Print and shaded views of the part. All mm, measured from the part's lowest x, y and z. A direction names the side the tool comes from. Round coordinates to 2 decimals unless told otherwise and drop trailing zeros. Loops run counter-clockwise (first coordinate to the right, second up) from the corner with the lowest first, then second, coordinate; pieces in that order, holes last. Notation, with made-up numbers: (72, 32) - (126, 32) arc R33 cw to (126, 66) - close; hole circle Ø9 at (16.25, -39). An arc over 180 degrees is marked (long way). Answer as a JSON object with one key per item and string values.
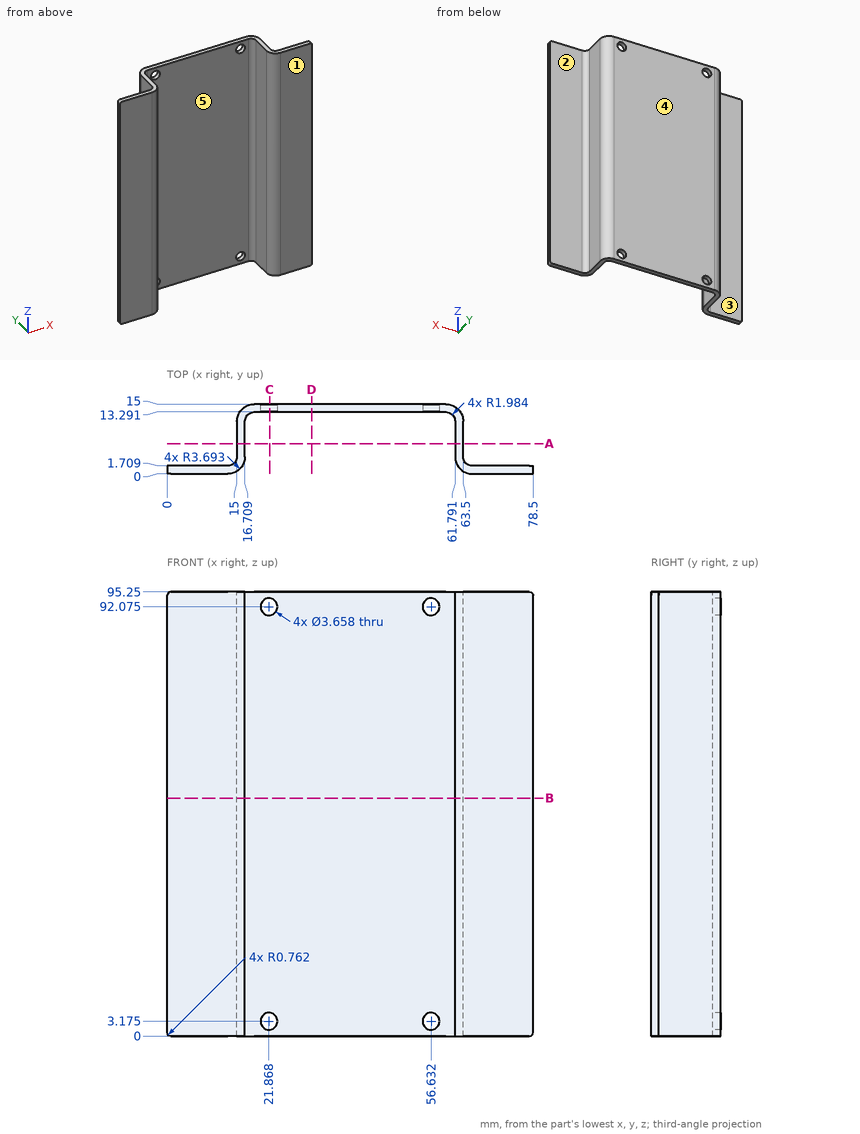
1) Slice it at A-A on y = 6.5. List the corners of the cut face in (x, z).
Values follow:
{"outline": "(15, 0) - (16.71, 0) - (16.71, 95.25) - (15, 95.25) - close; (61.79, 0) - (63.5, 0) - (63.5, 95.25) - (61.79, 95.25) - close"}
2) Two-plate mould, pull along X, no slides. Class the marked faces 4 and 5: pulls with the +X half, pulls with the -X half, needs draft (parallel to the pull), parting line crosses it, or undercut.
Values follow:
{"face 4": "needs draft", "face 5": "undercut"}
3) Slice it at D-D on x = 31. List the corners of the cut face in (y, z), then the cut area to 3 significant figures.
Values follow:
{"outline": "(13.29, 0) - (15, 0) - (15, 95.25) - (13.29, 95.25) - close", "area": "163 mm²"}
4) Tool access for the marked faces 1, 2 and 3: list every direction of +Z, -Z, +X, -X, +Y, -Y with a clear straight run to the whole face (end or side of a thin tool).
Values follow:
{"face 1": "+Z, -Z, +X, -X, -Y", "face 2": "+Z, -Z, +X, +Y", "face 3": "+Z, -Z, -X, +Y"}
5) Slice it at C-C on x = 22. List the corners of the cut face in (y, z).
Values follow:
{"outline": "(13.29, 0) - (15, 0) - (15, 1.35) - (13.29, 1.35) - close; (13.29, 5) - (15, 5) - (15, 90.25) - (13.29, 90.25) - close; (13.29, 93.9) - (15, 93.9) - (15, 95.25) - (13.29, 95.25) - close"}
6) Probe probe 1 along X at (y, z) = (5, 26); probe 2 along Y at (x, z) = (40, 49); probe 3 along Y at (x, z) = (13, 66.5). List the from-to ranges inside material, lowest first.
Values follow:
{"probe 1": "15 to 16.71, 61.79 to 63.5", "probe 2": "13.29 to 15", "probe 3": "0 to 1.71"}
7) Slice it at B-B on z = 51. List the corners of the cut face in (x, y).
Values follow:
{"outline": "(0, 0) - (13.02, 0) arc R3.69 ccw to (16.71, 3.69) - (16.71, 11.31) arc R1.98 cw to (18.69, 13.29) - (59.81, 13.29) arc R1.98 cw to (61.79, 11.31) - (61.79, 3.69) arc R3.69 ccw to (65.48, 0) - (78.5, 0) - (78.5, 1.71) - (65.48, 1.71) arc R1.98 cw to (63.5, 3.69) - (63.5, 11.31) arc R3.69 ccw to (59.81, 15) - (18.69, 15) arc R3.69 ccw to (15, 11.31) - (15, 3.69) arc R1.98 cw to (13.02, 1.71) - (0, 1.71) - close"}
8) Drop flat-ended pins along their axis: P1, Ø2, axis at y = 4, z = 26.5, coming from the -X side (1 decimal); P2, Ø2.5, axis at y = 7, z = 50, coming from the -X side; P3, Ø1.5, axis at y = 5.5, z = 61.5, coming from the +X side. Give the stop position or say it passes through.
Values follow:
{"P1": "x = 14.9", "P2": "x = 15", "P3": "x = 63.5"}
